Could you check a few things on this model? Use its own coordinates, in mm. A direction names the side the tool comes from. Round coordinates to 2 decimals unless told otherwise and drop trailing zeros. Order: outer loops, then holes, each group sorted by start corner. A loop starts at its lowest first (then second) coordinate and runs counter-clockwise, first axis right, second up.
```python
from build123d import *

# Parameters (mm, degrees)
SKETCH1_R           = 3.25
BOSS_EXTRUDE1_DEPTH = 3
SKETCH2_W           = 10
SKETCH2_H           = 600
BOSS_EXTRUDE2_DEPTH = 27
FILLET1_R           = 10


with BuildPart() as part:
    # Sketch1 → Boss-Extrude1 (new body)
    with BuildSketch(Plane.XY):
        Polygon((125, -300), (125, 300), (165, 300), (165, -300), (150, -300), align=None)
        with Locations((150, 270)):
            Circle(SKETCH1_R, mode=Mode.SUBTRACT)
        with Locations((150, 180)):
            Circle(SKETCH1_R, mode=Mode.SUBTRACT)
        with Locations((150, 90)):
            Circle(SKETCH1_R, mode=Mode.SUBTRACT)
        with Locations((150, 0)):
            Circle(SKETCH1_R, mode=Mode.SUBTRACT)
        with Locations((150, -90)):
            Circle(SKETCH1_R, mode=Mode.SUBTRACT)
        with Locations((150, -180)):
            Circle(SKETCH1_R, mode=Mode.SUBTRACT)
        with Locations((150, -270)):
            Circle(SKETCH1_R, mode=Mode.SUBTRACT)
    extrude(amount=BOSS_EXTRUDE1_DEPTH)

    # Sketch2 → Boss-Extrude2 (add)
    with BuildSketch(Plane.XY.offset(3)):
        with Locations((130, 0)):
            Rectangle(SKETCH2_W, SKETCH2_H)
    extrude(amount=BOSS_EXTRUDE2_DEPTH)

    # Fillet1
    fillet1_edges = [part.edges().sort_by_distance(p)[0] for p in [
        (135, 0, 3),
    ]]
    fillet(fillet1_edges, radius=FILLET1_R)


solid = part.part
```
Q1. I need wall thicknesses on L1, parallel to X at y = -180, z = 1.55; L2, parallel to Z at x = 162.5, y = -74.5; L3, parallel to X at y = 114.5, z = 24.25. Which ranges of each line are inside material? Lowest first, please.
Q2. Imagine slicing it at B-B, the plane z = 18.25. Please give me the cut outline in (x, y).
Q3. For P1, Ø1, axis at y = 149.5, z = 11, coming from the +X side; P2, Ø13.5, axis at y = -70, z = 25.5, coming from the +X side; P3, Ø1, axis at x = 141, y = 47, coming from the +Z side; P4, Ø4, axis at x = 150, y = 0, coming from the +Z side, each with a flat end and sliding along its axis, tell me the tip position at first contact or that it passes through.
Q4. Imagine slicing it at A-A, the plane y = 231.5. Please give me the cut outline in (x, z), then the cut area to 3 significant figures.
Q5. For faces 1 (the flat face through (155, 4, 3)), 2 (the flat face through (145, 4, 0)), which set-ups out of +Z, -Z, +X, -X, +Y, -Y let a thin tool reach every point of the face, with its end or its side?
Filled in:
1. L1: x = 125 to 146.75, 153.25 to 165
1. L2: z = 0 to 3
1. L3: x = 125 to 135
2. outline: (125, -300) - (135, -300) - (135, 300) - (125, 300) - close
3. P1: stops at x = 135.32
3. P2: stops at x = 135
3. P3: stops at z = 4.07
3. P4: passes through
4. outline: (125, 0) - (165, 0) - (165, 3) - (145, 3) arc R10 cw to (135, 13) - (135, 30) - (125, 30) - close
4. area: 411 mm2
5. face 1: +Z, +X, +Y, -Y
5. face 2: -Z, +X, -X, +Y, -Y
